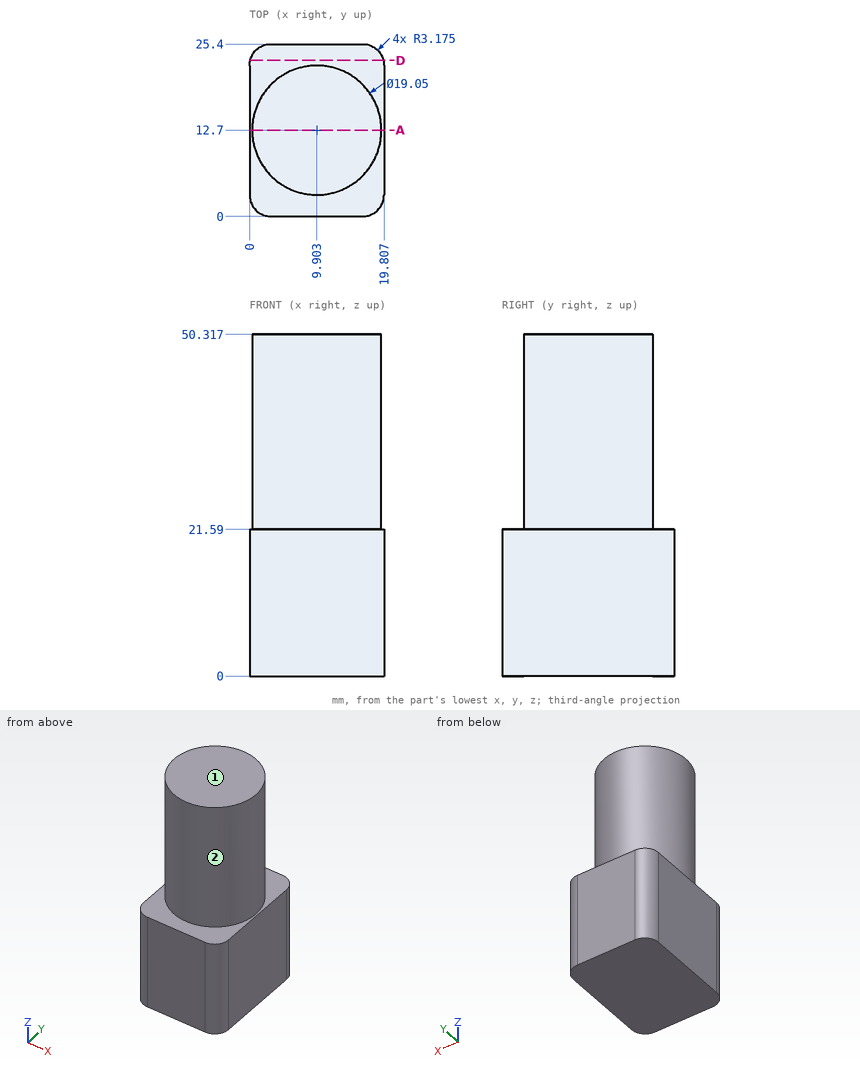
Check sheet for the drawn part. Datum: minimum x, y, z corner. Units: mm. A direction names the side the tool comes from. Round coordinates to 2 decimals unless told otherwise and drop trailing zeros. Write each loop counter-clockwise with the first axis right and the second up, starting at its lowest first coordinate (ties: lowest second). Pieces come first, ordered by that corner, then holes. Notation, with made-up numbers: (61, -4.5) -> (67, -4.5) arc R15 ccw to (67, 11.5) -> close; hole circle Ø8 at (69, 46). An arc over 180 degrees is marked (long way). One line per item, written item: value. Start each with the question number.
(1) Cross-section at D-D, the plane y = 23. Record the cut outline in (x, z).
(2) Scan lines: line 1 (Z direction, x = 19, y = 7); line 2 (Y direction, x = 18.25, z = 26); line 3 (X direction, y = 10.5, z = 48) (1 decimal). Record each from-to range of solid material in increasing order. Write a range as [from, to].
(3) Go/stop test with flat-tipped pins: pin 1 Ø3 at (x, z) = (6, 26) entering from +Y; pin 2 Ø3 at (y, z) = (15, 39.5) entering from -X; pin 3 Ø5 at (x, z) = (8, 26) entering from +Y (3 decimals). Record where each tip stops, or that it passes through.
(4) Cross-section at A-A, the plane y = 12.7. Record the cut outline in (x, z), and give its area (3 significant figures).
(5) Access from +Z, -Z, +X, -X, +Y, -Y to the whole of each face (thin tool, end or side, straight path). Record for the marked faces 1 and 2.
Answer:
1. outline: (0.1, 0) -> (19.71, 0) -> (19.71, 21.59) -> (0.1, 21.59) -> close
2. line 1: [0, 21.59]
2. line 2: [8.11, 17.29]
2. line 3: [0.6, 19.2]
3. pin 1: y = 21.92
3. pin 2: x = 0.41
3. pin 3: y = 22.225
4. outline: (0, 0) -> (19.81, 0) -> (19.81, 21.59) -> (19.43, 21.59) -> (19.43, 50.32) -> (0.38, 50.32) -> (0.38, 21.59) -> (0, 21.59) -> close
4. area: 975 mm²
5. face 1: +Z, +X, -X, +Y, -Y
5. face 2: +Z
